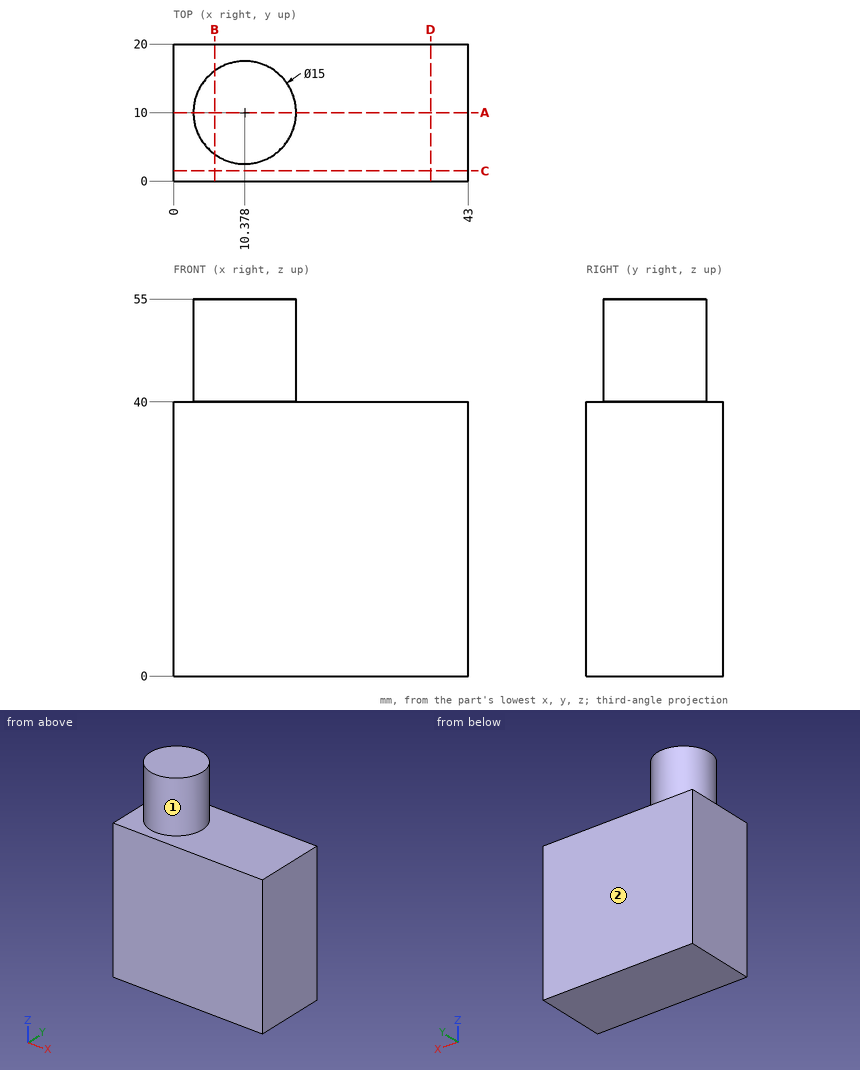
Geometry check sheet. Reference: drawing and pictorial views, mm from the part's lowest x, y, z. A direction names the side the tool comes from. Round coordinates to 2 decimals unless told otherwise and drop trailing zeros. Loops run counter-clockwise (first coordinate to the right, second up) from the corner with the lowest first, then second, coordinate; pieces in that order, holes last. Notation, with made-up numbers: (15.25, 60.25) - (74.25, 60.25) arc R19 ccw to (74.25, 73.25) - close; hole circle Ø2 at (66.25, 44.5). An arc over 180 degrees is marked (long way). Answer in a Markdown table with one row per item. Add a question column.
Q1. Section check D-D on x = 37.5. Enter the section's corners in (y, z), plus the area to 3 significant figures.
Q2. Material ranges on line 1 (Z direction, x = 27.5, y = 11.75); line 2 (X direction, y = 12.25, z = 44.5); line 3 (X direction, y = 7, z = 47.5), recorded low to high.
Q3. Gauge pin test, flat ends, axial feed: pin 1 (5 mm diameter, centred on y = 15.5, z = 45, fed in from +X); pin 2 (6 mm diameter, centred on x = 24, y = 5, fed in from +Z). Record the tip position at first contact, or that the pin passes through.
Q4. Section check A-A on y = 10. Enter the section's corners in (x, z).
Q5. Section check B-B on x = 6. Enter the section's corners in (y, z).
Q6. Tool access check on the marked faces 1 and 2. Record the directions out of +Z, -Z, +X, -X, +Y, -Y that give a thin tool (end or side, any length) a straight path to the whole face; none if there is none.
Q7. Section check C-C on y = 1.5. Enter the section's corners in (x, z), plus the area to 3 significant figures.
Found:
| question | item | result |
|---|---|---|
| 1 | outline | (0, 0) - (20, 0) - (20, 40) - (0, 40) - close |
| 1 | area | 800 mm² |
| 2 | line 1 | z = 0 to 40 |
| 2 | line 2 | x = 3.22 to 17.53 |
| 2 | line 3 | x = 3.5 to 17.25 |
| 3 | pin 1 | stops at x = 17.25 |
| 3 | pin 2 | stops at z = 40 |
| 4 | outline | (0, 0) - (43, 0) - (43, 40) - (17.88, 40) - (17.88, 55) - (2.88, 55) - (2.88, 40) - (0, 40) - close |
| 5 | outline | (0, 0) - (20, 0) - (20, 40) - (16.09, 40) - (16.09, 55) - (3.91, 55) - (3.91, 40) - (0, 40) - close |
| 6 | face 1 | +Z |
| 6 | face 2 | +Z, -Z, +X, -X, +Y |
| 7 | outline | (0, 0) - (43, 0) - (43, 40) - (0, 40) - close |
| 7 | area | 1,720 mm² |
